Autodesk Fusion 360 part; units mm, degrees
sketch "Sketch1" plane through (0, 0, 0) normal (0, 0, 1) x (1, 0, 0)
  line L0 (0, 50) -> (0, -40) construction
  line L1 (-50, 0) -> (45, 0) construction
  line L2 (-17.5, 27.5) -> (17.5, 27.5)
  line L3 (17.5, 27.5) -> (17.5, -27.5)
  line L4 (17.5, -27.5) -> (-17.5, -27.5)
  line L5 (-17.5, -27.5) -> (-17.5, 27.5)
  line L6 (-13, 23) -> (13, 23) construction
  line L7 (13, 23) -> (13, -23) construction
  line L8 (13, -23) -> (-13, -23) construction
  line L9 (-13, -23) -> (-13, 23) construction
  circle A0 centre (-13, 23) radius 2.5
  circle A1 centre (-13, 23) radius 1
  line L10 (-13, 23) -> (-2, 23) construction
  line L11 (-2, 23) -> (-2, 18) construction
  line L12 (-2, 18) -> (-13, 18) construction
  line L13 (-13, 18) -> (-13, 23) construction
  circle A2 centre (-2, 18) radius 2
  dimension "d1" = 35
  dimension "d2" = 55
  dimension "d3" = 17.5
  dimension "d4" = 27.5
  dimension "d5" = 26
  dimension "d6" = 46
  dimension "d7" = 13
  dimension "d8" = 23
  dimension "d9" = 5
  dimension "d10" = 2
  dimension "d63" = 11
  dimension "d64" = 5
  dimension "d65" = 4
extrude "Extrude1" add sketch "Sketch1" along normal blind 4 contours A0 makes body 1
pattern_linear "R-Pattern1" count 2 spacing 46 along (0, -1, 0) count 2 spacing 26 along (1, 0, 0) of bodies 1 makes body 2 at (15.4969, 22.8754, 2.6667) makes body 3 at (-10.5031, -23.1246, 2.6667) makes body 4 at (15.4969, -23.1246, 2.6667)
extrude "Extrude2" add sketch "Sketch1" along normal blind 1.5 separate body contours L2 L3 L4 L5 | A2 makes body 5
sketch "Sketch2" plane through (0, -27.5, 0) normal (0, -1, 0) x (1, 0, 0)
  line L0 (-17.5, 0) -> (17.5, 0)
  line L1 (17.5, 0) -> (17.5, 1.5)
  line L2 (17.5, 1.5) -> (-17.5, 1.5)
  line L3 (-17.5, 1.5) -> (-17.5, 0)
  line L4 (-17.5, 0) -> (17.5, 0)
  line L5 (17.5, 0) -> (17.5, 19.5)
  line L6 (17.5, 19.5) -> (-17.5, 19.5)
  line L7 (-17.5, 19.5) -> (-17.5, 0)
  line L8 (-19, 21) -> (19, 21)
  line L9 (19, 21) -> (19, 0)
  line L10 (19, 0) -> (-19, 0)
  line L11 (-19, 0) -> (-19, 21)
  line L12 (17.5, 0) -> (-17.5, 0)
  line L13 (-17.5, 0) -> (17.5, 0)
  line L14 (17.5, 0) -> (17.5, -17)
  line L15 (17.5, -17) -> (-17.5, -17)
  line L16 (-17.5, -17) -> (-17.5, 0)
  line L17 (-19, 0) -> (19, 0)
  line L18 (19, 0) -> (19, -18.5)
  line L19 (19, -18.5) -> (-19, -18.5)
  line L20 (-19, -18.5) -> (-19, 0)
  line L21 (-20.5, -19.25) -> (20.5, -19.25)
  line L22 (20.5, -19.25) -> (20.5, 21.75)
  line L23 (20.5, 21.75) -> (-20.5, 21.75)
  line L24 (-20.5, 21.75) -> (-20.5, -19.25)
  line L25 (-19, -17.75) -> (19, -17.75)
  line L26 (19, -17.75) -> (19, 20.25)
  line L27 (19, 20.25) -> (-19, 20.25)
  line L28 (-19, 20.25) -> (-19, -17.75)
  line L29 (-21.5, -20.25) -> (21.5, -20.25)
  line L30 (21.5, -20.25) -> (21.5, 22.75)
  line L31 (21.5, 22.75) -> (-21.5, 22.75)
  line L32 (-21.5, 22.75) -> (-21.5, -20.25)
  line L33 (-18.5, 15) -> (-18.5, 26)
  line L34 (14.5, 15) -> (14.5, 25)
  line L35 (-23.5, -22.25) -> (23.5, -22.25)
  line L36 (23.5, -22.25) -> (23.5, 24.75)
  line L37 (23.5, 24.75) -> (-23.5, 24.75)
  line L38 (-23.5, 24.75) -> (-23.5, -22.25)
  line L39 (-14.5, 15) -> (-14.5, 32)
  dimension "d19" = 35
  dimension "d20" = 19.5
  dimension "d22" = 1.5
  dimension "d23" = 1.5
  dimension "d24" = 1.5
  dimension "d25" = 17
  dimension "d83" = 1.5
  dimension "d86" = 3
  dimension "d88" = 2.25
  dimension "d90" = 2.25
  dimension "d91" = 1.5
  dimension "d92" = 1.5
  dimension "d93" = 1.5
  dimension "d94" = 1.5
  dimension "d100" = 1
  dimension "d101" = 1
  dimension "d102" = 1
  dimension "d103" = 1
  dimension "d104" = 2
  dimension "d105" = 6
  dimension "d112" = 2
  dimension "d113" = 2
  dimension "d114" = 2
  dimension "d115" = 2
  dimension "d118" = 3
  dimension "d119" = 3
extrude "Extrude3" add sketch "Sketch2" against normal blind 55 contours L3 L6 L7 L10 L11 L17 L27 L28 L39 | L10 L14 L15 L16 L17 L18 L20 L25 L26 L28 | L1 L5 L6 L9 L10 L17 L26 L27 L34 | L8 L11 L27 L33 | L18 L19 L20 L25 | L8 L9 L27 L34 | L6 L27 L34 L39 | L8 L27 L33 L39 | L8 L27 L34 L39 bodies 5
extrude "Extrude4" add sketch "Sketch2" along normal blind 1.5 separate body contours L0 L4 L10 L12 L13 L14 L15 L16 L17 makes body 6
extrude "Extrude5" add sketch "Sketch2" along normal blind 21.5 contours L10 L14 L15 L16 L17 L18 L20 L25 L26 L28 | L18 L19 L20 L25 bodies 5 6
sketch "Sketch3" plane through (0, -49, 0) normal (0, -1, 0) x (1, 0, 0)
  line L0 (17.5, 0) -> (17.5, -17)
  line L1 (17.5, -17) -> (-17.5, -17)
  line L2 (-17.5, -17) -> (-17.5, 0)
  line L3 (-17.5, 0) -> (-19, 0)
  line L4 (-19, 0) -> (-19, -18.5)
  line L5 (-19, -18.5) -> (19, -18.5)
  line L6 (19, -18.5) -> (19, 0)
  line L7 (19, 0) -> (17.5, 0)
  line L8 (-19, 0) -> (19, 0)
  line L9 (19, 0) -> (19, -18.5)
  line L10 (19, -18.5) -> (-19, -18.5)
  line L11 (-19, -18.5) -> (-19, 0)
  line L12 (-46.8165, -8.5) -> (11.8165, -8.5) construction
  line L13 (-17.5, -17) -> (-17.5, 0) construction
  line L14 (0, -10.2369) -> (0, -23.7631) construction
  line L15 (17.5, -17) -> (-17.5, -17) construction
  line L16 (-10.5, -1.75) -> (10.5, -1.75)
  line L17 (10.5, -1.75) -> (10.5, -15.25)
  line L18 (10.5, -15.25) -> (-10.5, -15.25)
  line L19 (-10.5, -15.25) -> (-10.5, -1.75)
  dimension "d32" = 21
  dimension "d33" = 13.5
  dimension "d34" = 10.5
  dimension "d35" = 6.75
extrude "Extrude6" add sketch "Sketch3" along normal blind 1.5 separate body makes body 7
sketch "Sketch4" plane through (0, 0, 4) normal (0, 0, 1) x (1, 0, 0)
  circle A0 centre (-13, 23) radius 1
  circle A1 centre (-13, 23) radius 2.5
extrude "Extrude8" add sketch "Sketch4" along normal blind 20 separate body contours A0 | A1 makes body 8
pattern_linear "R-Pattern2" count 2 spacing 46 along (0, -1, 0) count 2 spacing 26 along (1, 0, 0) of bodies 8 makes body 9 at (15.4969, 22.8754, 17.3333) makes body 10 at (-10.5031, -23.1246, 17.3333) makes body 11 at (15.4969, -23.1246, 17.3333)
combine "Combine1" operation cut target body 5 tool bodies 11 10 9 8
sketch "Sketch5" plane through (0, -27.5, 0) normal (0, -1, 0) x (1, 0, 0)
  line L0 (-19, 0) -> (-17.5, 0)
  line L1 (-17.5, 0) -> (-17.5, 21)
  line L2 (-17.5, 21) -> (-19, 21)
  line L3 (-19, 21) -> (-19, 0)
  line L4 (-19, 21) -> (19, 21)
  line L5 (17.5, 0) -> (19, 0)
  line L6 (19, 0) -> (19, 21)
  line L7 (19, 21) -> (17.5, 21)
  line L8 (17.5, 21) -> (17.5, 0)
  point P0 (-19, 0)
  point P1 (17.5, 0)
extrude "Extrude9" add sketch "Sketch5" along normal blind 23 bodies 7 5
sketch "Sketch6" plane through (0, 0, 0) normal (0, 0, 1) x (1, 0, 0)
  line L0 (-17.5, -27.5) -> (-17.5, -29)
  line L1 (-17.5, -29) -> (17.5, -29)
  line L2 (17.5, -29) -> (17.5, -27.5)
  line L3 (17.5, -27.5) -> (-17.5, -27.5)
extrude "Extrude10" add sketch "Sketch6" along normal blind 1.5 bodies 7
sketch "Sketch7" plane through (0, -29, 0) normal (0, -1, 0) x (1, 0, 0)
  line L0 (-17.5, -17) -> (17.5, -17)
  line L1 (17.5, -17) -> (17.5, 1.5)
  line L2 (17.5, 1.5) -> (-17.5, 1.5)
  line L3 (-17.5, 1.5) -> (-17.5, -17)
  circle A0 centre (-15, -7) radius 2
  dimension "d50" = 4
extrude "Extrude11" cut sketch "Sketch7" against normal blind 3 contours A0 bodies 7
sketch "Sketch8" plane through (0, 0, 0) normal (0, 0, 1) x (1, 0, 0)
  line L0 (-17.5, -49) -> (-17.5, -50.5)
  line L1 (-17.5, -50.5) -> (17.5, -50.5)
  line L2 (17.5, -50.5) -> (17.5, -49)
  line L3 (17.5, -49) -> (-17.5, -49)
extrude "Extrude12" add sketch "Sketch8" along normal blind 3 bodies 7
extrude "Extrude13" add sketch "Sketch2" along normal blind 1.5 contours L3 L6 L7 L10 L11 L17 L27 L28 L39 | L1 L5 L6 L9 L10 L17 L26 L27 L34 | L8 L11 L27 L33 | L8 L9 L27 L34 | L6 L27 L34 L39 | L8 L27 L33 L39 | L8 L27 L34 L39 bodies 7
combine "Combine2" operation add target body 7 tool bodies 4 3 2 1
extrude "Extrude14" add 1 faces at (12.4588, -23.1083, 1.5) along direction (0, 0, -1) blind 1.5 separate body on bodies 7 makes body 12
pattern_linear "R-Pattern3" count 2 spacing 46 along (0, 1, 0) count 2 spacing 26 along (1, 0, 0) of bodies 12 makes body 13 at (39.6617, -23.7498, 0.5) makes body 14 at (13.9988, 23.0498, 0.5) makes body 15 at (39.6617, 22.2502, 0.5)
combine "Combine3" operation cut target body 7 tool bodies 12 13 14 15
extrude "Extrude15" add sketch "Sketch1" along normal blind 20 separate body contours A2 makes body 16
pattern_linear "R-Pattern4" count 2 spacing 5 along (1, 0, 0) of bodies 16 makes body 17
move_body "Move1" bodies 16 17 to x (1, 0, 0) y (0, 1, 0) z (0, 0, 1) at (0, 0, 5)
combine "Combine4" operation cut target body 7 tool bodies 16 17
fillet "Fillet1" radius 1 2 edges at (-18.25, -50.5, 21) (18.25, -50.5, 21) on bodies 7
fillet "Fillet1" radius 1 1 edges at (0, -50.5, -18.5) on bodies 7
fillet "Fillet1" radius 1 2 edges at (19, -50.5, 1.25) (-19, -50.5, 1.25) on bodies 7
extrude "Extrude23" add sketch "Sketch2" along normal blind 10 separate body contours L8 L9 L11 L18 L19 L20 L21 L22 L23 L24 L26 L28 L33 L34 | L8 L11 L27 L33 | L18 L19 L20 L25 | L8 L9 L27 L34 makes body 18
extrude "Extrude24" add sketch "Sketch2" against normal blind 3 contours L8 L9 L11 L18 L19 L20 L21 L22 L23 L24 L26 L28 L33 L34 | L8 L11 L27 L33 | L18 L19 L20 L25 | L8 L9 L27 L34 bodies 18
extrude "Extrude25" add sketch "Sketch2" against normal blind 3 contours L21 L22 L23 L24 L29 L30 L31 L32 L33 L34 bodies 18
extrude "Extrude26" add sketch "Sketch2" against normal blind 20 contours L31 L33 L37 L39 | L29 L30 L31 L32 L33 L34 L35 L36 L37 L38 | L31 L34 L37 L39 bodies 18
extrude "Extrude27" cut sketch "Sketch2" against normal blind 15 contours L31 L33 L37 L39 | L31 L34 L37 L39 bodies 18
hidden bodies 18
equation "d3 = d1 / 2"
equation "d4 = d2 / 2"
equation "d7 = d5 / 2"
equation "d8 = d6 / 2"
equation "d22 = Linear Dimension-4"
equation "d23 = Linear Dimension-5"
equation "d24 = Linear Dimension-6"
equation "d26 = -d2"
equation "d30 = 20 mm + e"
equation "d34 = d32 / 2"
equation "d35 = ( d33 / 2 )"
equation "d46 = 20 mm + 2 * e"
equation "d83 = Linear Dimension-8"
equation "e2 = 2 mm"
equation "d86 = ( L - d19 ) / 2"
equation "d88 = ( L - d20 - d25 ) / 2"
equation "d90 = ( L - d20 - d25 ) / 2"
equation "d91 = Linear Dimension-13"
equation "d92 = Linear Dimension-14"
equation "d93 = Linear Dimension-15"
equation "d94 = Linear Dimension-16"
equation "LB = 43 mm"
equation "d100 = ( LB - L ) / 2"
equation "d101 = ( LB - L ) / 2"
equation "d102 = ( LB - L ) / 2"
equation "d103 = ( LB - L ) / 2"
equation "d112 = e2"
equation "d113 = e2"
equation "d114 = e2"
equation "d115 = e2"
equation "d119 = ( L - d19 ) / 2"
Geometry check sheet. Reference: the model listing, model coordinates, mm. A direction names the side the tool comes from. Coordinates: 2 decimals unless noted, no trailing zeros. Loops run counter-clockwise (first coordinate to the right, second up) from the corner with the lowest first, then second, coordinate; pieces in that order, holes last. Notation, with made-up numbers: (82.5, 58) - (139.5, 58) arc R4 ccw to (139.5, 63) - close; hole circle Ø4 at (51.5, 34). An arc over 180 degrees is marked (long way). Use one line per item in the form item = value. Start each with the question number.
Item 1: Section check A-A, the plane y = 18. Enter the section's corners in (x, z).
Item 2: Section check C-C, the plane z = 5.5. Enter the section's corners in (x, y).
Item 3: Tool access check on faces 4 (the face through (0, -27.5, -8)), 5 (the face through (-19, -10, 2)), 6 (the face through (0, -39, -17)), 7 (the face through (-12, -24, 4)), 8 (the face through (12.67, -25.48, 2.73)). Record the directions out of +Z, -Z, +X, -X, +Y, -Y that give a thin tool (end or side, any length) a straight path to the whole face; none if there is none.
Item 4: Section check D-D, the plane y = -4. Enter the section's corners in (x, z).
Item 5: Gauge pin test, flat ends, axial feed: pin 1 (0.8 mm diameter, centred on x = 0, y = -49.5, fed in from +Z); pin 2 (1 mm diameter, centred on x = 14.5, z = -10, fed in from +Y); pin 3 (4 mm diameter, centred on x = 10.5, z = 7.5, fed in from +Y); pin 4 (0.8 mm diameter, centred on x = -5.5, z = 20, fed in from -Y). Record the tip position at first contact, or that the pin passes through.
Item 6: Mould release check, pull along Z, two halves, no side actions. Record for faces 1 (the face through (3, 16, 20)), 2 (the face through (14, -24, 4)), 3 (the face through (-17.5, -20, 6)): +Z half, -Z half, draft (parallel to the pull), parting line (faces both ways), or undercut.
Item 7: Section check B-B, the plane x = 7.5. Enter the section's corners in (y, z).
Item 8: Thickness scan on probe 1 along X at (y, z) = (-23, 20); probe 2 along Z at (x, y) = (10, -6.5); probe 3 along Y at (x, z) = (-13, 20.3). Record the ranges inside material, lowest first.
Computed:
q1.outline = (-19, -18.5) - (19, -18.5) - (19, 21) - (5, 21) - (5, 19.5) - (17.5, 19.5) - (17.5, 1.5) - (-17.5, 1.5) - (-17.5, 19.5) - (-4, 19.5) - (-4, 21) - (-19, 21) - close; (0, 19.5) - (1, 19.5) - (1, 21) - (0, 21) - close; hole (-17.5, -17) - (17.5, -17) - (17.5, 0) - (-17.5, 0) - close
q2.outline = (-19, -49.5) arc R1 ccw to (-18, -50.5) - (-17.5, -50.5) - (-17.5, 27.5) - (-19, 27.5) - close; (17.5, -50.5) - (18, -50.5) arc R1 ccw to (19, -49.5) - (19, 27.5) - (17.5, 27.5) - close
q3.face_4 = +Y
q3.face_5 = +Z, -Z, -X, +Y, -Y
q3.face_6 = +Z
q3.face_7 = +Z, +Y, -Y
q3.face_8 = none
q4.outline = (-19, -18.5) - (19, -18.5) - (19, 21) - (-19, 21) - close; hole (-17.5, -17) - (17.5, -17) - (17.5, 0) - (-17.5, 0) - close; hole (-17.5, 1.5) - (17.5, 1.5) - (17.5, 19.5) - (-17.5, 19.5) - close
q5.pin_1 = 3
q5.pin_2 = -27.5
q5.pin_3 = through
q5.pin_4 = -29
q6.face_1 = draft
q6.face_2 = +Z half
q6.face_3 = undercut
q7.outline = (-50.5, -17.5) arc R1 ccw to (-49.5, -18.5) - (27.5, -18.5) - (27.5, -17) - (-27.5, -17) - (-27.5, 0) - (27.5, 0) - (27.5, 1.5) - (-29, 1.5) - (-29, -17) - (-49, -17) - (-49, -15.25) - (-50.5, -15.25) - close; (-50.5, -1.75) - (-49, -1.75) - (-49, 3) - (-50.5, 3) - close; (-29, 19.5) - (27.5, 19.5) - (27.5, 21) - (-29, 21) - close
q8.probe_1 = -19 to -15.5, -10.5 to 10.5, 15.5 to 19
q8.probe_2 = -18.5 to -17, 0 to 1.5, 19.5 to 21
q8.probe_3 = -29 to -25.5, -20.5 to 20.5, 25.5 to 27.5
